Can you work these out from the model? Positions are in its coordinate system, mm. Face numbers are marked on the shaded views. A direction names the side the tool comes from. Round coordinates to 2 decimals unless told otherwise and drop trailing zeros. Loops run counter-clockwise (first coordinate to the right, second up) from the corner with the lowest first, then second, coordinate; pieces in that order, holes last.
(1) I want a section at D-D on x = 10.5. Write out the boundary of the cut face in (y, z), plus the area to 3 significant figures.
(2) If I drill on line 1 along Z through (x, y) = (-7.5, 2.95); line 2 along X through (y, z) = (1.35, 14.8); line 3 along Z through (x, y) = (16, 85), over which ranges is the centre line in solid material (lowest first)?
(3) Will these pins go through, and if not, where does the flat tip stop? pin 1 Ø1.5 at (x, z) = (13.5, -15.5) entering from +Y; pin 2 Ø8 at (y, z) = (63.5, -4) entering from +X; pin 3 Ø5 at (x, y) = (14, 83.5) entering from -Z; pin 4 Ø6.5 at (x, y) = (15.41, 98.67) entering from +Z.
(4) I want a section at C-C on y = 79.03. Write out the boundary of the cut face in (x, z), plus the area to 4 significant figures.
(5) Which directions (+Z, -Z, +X, -X, +Y, -Y) give clear straight access to the entire face, cutting with the end or side of a thin tool? Please do the marked faces 1, 2 and 3.
(6) Thinking about a two-plate mould opening in Y: for the marked faces 4, 5 and 6, which applies, released by +Y, released by -Y, zero draft, split by the parting line, or undercut?
(7) I want a section at B-B on z = -14.8. Write out the boundary of the cut face in (x, y), plus the area to 3 significant figures.
(8) I want a section at A-A on x = 15.41. Give the number of separate pieces and of enclosed holes in the cut face, plus the area to 3 significant figures.
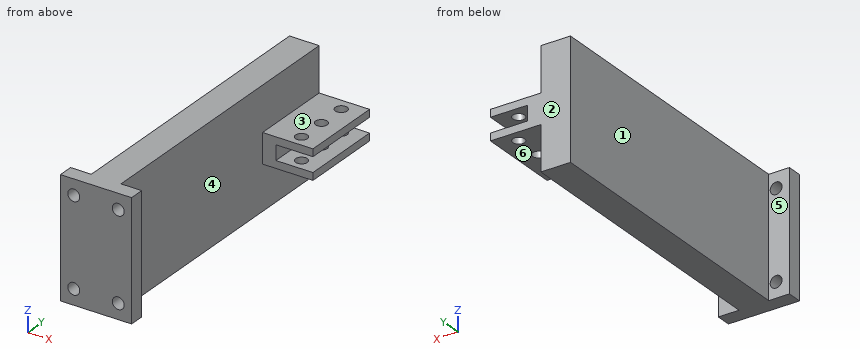
from build123d import *

# Parameters (mm, degrees)
SKETCH_1_W          = 24
SKETCH_1_H          = 40
SKETCH_1_R          = 2
EXTRUDE_1_DEPTH     = 5
EXTRUDE_5_DEPTH     = 98
SKETCH_10_W         = 10
SKETCH_10_H         = 28
EXTRUDE_6_DEPTH     = 18.5
SKETCH_12_R         = 2
CUT_EXTRUDE_4_DEPTH = 24.25
SKETCH_13_W         = 12
SKETCH_13_H         = 28
CUT_EXTRUDE_5_DEPTH = 2
SKETCH_14_W         = 2
SKETCH_14_H         = 4
CUT_EXTRUDE_6_DEPTH = 34
SKETCH_15_W         = 12.5
SKETCH_15_H         = 0.5
CUT_EXTRUDE_7_DEPTH = 34


with BuildPart() as part:
    # 草图1 → 凸台-拉伸1 (new body)
    with BuildSketch(Plane(origin=(0, 0, 0), x_dir=(1, 0, 0), z_dir=(0, 1, 0))):
        Rectangle(SKETCH_1_W, SKETCH_1_H)
        with Locations((7.5, -14.8)):
            Circle(SKETCH_1_R, mode=Mode.SUBTRACT)
        with Locations((-7.5, -14.8)):
            Circle(SKETCH_1_R, mode=Mode.SUBTRACT)
        with Locations((-7.5, 14.8)):
            Circle(SKETCH_1_R, mode=Mode.SUBTRACT)
        with Locations((7.5, 14.8)):
            Circle(SKETCH_1_R, mode=Mode.SUBTRACT)
    extrude(amount=EXTRUDE_1_DEPTH)

    # 草图8 → 凸台-拉伸5 (add)
    with BuildSketch(Plane(origin=(0, 5, 0), x_dir=(1, 0, 0), z_dir=(0, 1, 0))):
        Polygon((-5, 0), (-5, -20), (5, -20), (5, 20), (-5, 20), align=None)
    extrude(amount=EXTRUDE_5_DEPTH)

    # 草图10 → 凸台-拉伸6 (add)
    with BuildSketch(Plane(origin=(5, 0, 0), x_dir=(0, 0, -1), z_dir=(1, 0, 0))):
        with Locations((0, 89)):
            Rectangle(SKETCH_10_W, SKETCH_10_H)
    extrude(amount=EXTRUDE_6_DEPTH)

    # 草图12 → 切除-拉伸4 (cut, symmetric)
    with BuildSketch(Plane(origin=(0, 0, -5), x_dir=(-1, 0, 0), z_dir=(0, 0, -1))):
        with Locations((-15.41, 98.67)):
            Circle(SKETCH_12_R)
        with Locations((-15.41, 88.85)):
            Circle(SKETCH_12_R)
        with Locations((-15.41, 79.03)):
            Circle(SKETCH_12_R)
    extrude(amount=CUT_EXTRUDE_4_DEPTH, both=True, mode=Mode.SUBTRACT)

    # 草图13 → 切除-拉伸5 (cut, symmetric)
    with BuildSketch(Plane.XY):
        with Locations((17.5, 89)):
            Rectangle(SKETCH_13_W, SKETCH_13_H)
    extrude(amount=CUT_EXTRUDE_5_DEPTH, both=True, mode=Mode.SUBTRACT)

    # 草图14 → 切除-拉伸6 (cut)
    with BuildSketch(Plane(origin=(0, 103, 0), x_dir=(1, 0, 0), z_dir=(0, 1, 0))):
        with Locations((10.5, 0)):
            Rectangle(SKETCH_14_W, SKETCH_14_H)
        Polygon((22, 5), (23.5, 5), (23.5, 2), (23.5, -2), (23.5, -5), (22, -5), (22, -2.5), (22, 2.5), align=None)
    extrude(amount=-CUT_EXTRUDE_6_DEPTH, mode=Mode.SUBTRACT)

    # 草图15 → 切除-拉伸7 (cut)
    with BuildSketch(Plane(origin=(0, 103, 0), x_dir=(1, 0, 0), z_dir=(0, 1, 0))):
        with Locations((15.75, 2.25)):
            Rectangle(SKETCH_15_W, SKETCH_15_H)
        with Locations((15.75, -2.25)):
            Rectangle(SKETCH_15_W, SKETCH_15_H)
    extrude(amount=-CUT_EXTRUDE_7_DEPTH, mode=Mode.SUBTRACT)


solid = part.part
Filled sheet:
1. outline: (0, -20) - (5, -20) - (5, 20) - (0, 20) - close; (75, -5) - (103, -5) - (103, -2.5) - (75, -2.5) - close; (75, 2.5) - (103, 2.5) - (103, 5) - (75, 5) - close
1. area: 340 mm2
2. line 1: z = -20 to -16.8, -12.8 to 12.8, 16.8 to 20
2. line 2: x = -12 to -9.5, -5.5 to 5.5, 9.5 to 12
2. line 3: z = -5 to -2.5, 2.5 to 5
3. pin 1: passes through
3. pin 2: stops at x = 5
3. pin 3: stops at z = -5
3. pin 4: stops at z = 5
4. outline: (-5, -20) - (5, -20) - (5, -5) - (13.41, -5) - (13.41, -2.5) - (9.5, -2.5) - (9.5, 2.5) - (13.41, 2.5) - (13.41, 5) - (5, 5) - (5, 20) - (-5, 20) - close; (17.41, -5) - (22, -5) - (22, -2.5) - (17.41, -2.5) - close; (17.41, 2.5) - (22, 2.5) - (22, 5) - (17.41, 5) - close
4. area: 487.5 mm2
5. face 1: +Z, -Z, -X, +Y
5. face 2: +Z, -Z, +X, -X, +Y
5. face 3: +Z, +X, +Y
6. face 4: undercut
6. face 5: released by +Y
6. face 6: zero draft
7. outline: (-12, 0) - (-9.5, 0) - (-9.5, 5) - (-12, 5) - close; (-5.5, 0) - (5.5, 0) - (5.5, 5) - (5, 5) - (5, 103) - (-5, 103) - (-5, 5) - (-5.5, 5) - close; (9.5, 0) - (12, 0) - (12, 5) - (9.5, 5) - close
7. area: 1,060 mm2
8. separate pieces: 8
8. enclosed holes: 0
8. area: 80.0 mm2
